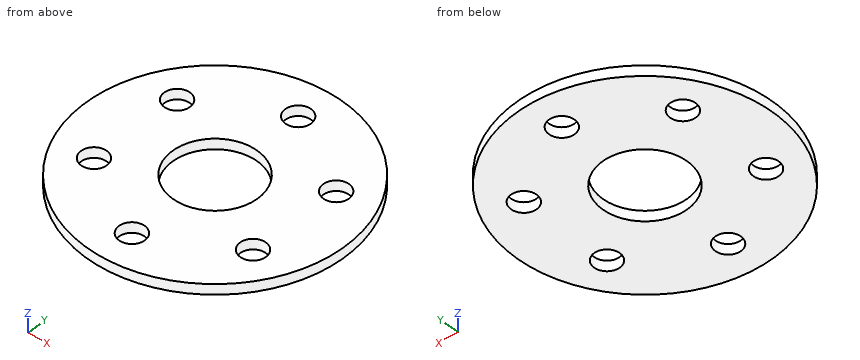
```python
from build123d import *

# Parameters (mm, degrees)
SKETCH1_R           = 25
SKETCH1_R_2         = 8.25
SKETCH1_R_3         = 2.5
BOSS_EXTRUDE1_DEPTH = 1


with BuildPart() as part:
    # Sketch1 (on Front Plane) → Boss-Extrude1 (new, symmetric)
    with BuildSketch(Plane.XY):
        Circle(SKETCH1_R)
        Circle(SKETCH1_R_2, mode=Mode.SUBTRACT)
        with Locations((0, 18)):
            Circle(SKETCH1_R_3, mode=Mode.SUBTRACT)
        with Locations((15.588457268, 9)):
            Circle(SKETCH1_R_3, mode=Mode.SUBTRACT)
        with Locations((15.588457268, -9)):
            Circle(SKETCH1_R_3, mode=Mode.SUBTRACT)
        with Locations((0, -18)):
            Circle(SKETCH1_R_3, mode=Mode.SUBTRACT)
        with Locations((-15.588457268, -9)):
            Circle(SKETCH1_R_3, mode=Mode.SUBTRACT)
        with Locations((-15.588457268, 9)):
            Circle(SKETCH1_R_3, mode=Mode.SUBTRACT)
    extrude(amount=BOSS_EXTRUDE1_DEPTH, both=True)


solid = part.part
```
Build history of the part. All positions in model axes, mm. Round coordinates to 2 decimals unless told otherwise and drop trailing zeros. Loops run counter-clockwise (first coordinate to the right, second up) from the corner with the lowest first, then second, coordinate; pieces in that order, holes last.
Item 1: Saw through at B-B (x = 0). List the corners of the cut face in (y, z), then the cut area to 3 significant figures.
Item 2: Saw through at C-C (x = -5). List the corners of the cut face in (y, z).
Item 3: Saw through at D-D (y = -9). List the corners of the cut face in (x, z), then the cut area to 3 significant figures.
Item 4: Saw through at A-A (y = 0). List the corners of the cut face in (x, z).
Item 5: Drill centre lines: line 1 along Y through (x, z) = (0, -0.4); line 2 along X through (y, z) = (-17.5, 0.55); line 3 along Y through (x, z) = (-5, 0.25). Where is each one in solid material? Low to high.
Worked answers:
1. outline: (-25, -1) - (-20.5, -1) - (-20.5, 1) - (-25, 1) - close; (-15.5, -1) - (-8.25, -1) - (-8.25, 1) - (-15.5, 1) - close; (8.25, -1) - (15.5, -1) - (15.5, 1) - (8.25, 1) - close; (20.5, -1) - (25, -1) - (25, 1) - (20.5, 1) - close
1. area: 47.0 mm2
2. outline: (-24.49, -1) - (-6.56, -1) - (-6.56, 1) - (-24.49, 1) - close; (6.56, -1) - (24.49, -1) - (24.49, 1) - (6.56, 1) - close
3. outline: (-23.32, -1) - (-18.09, -1) - (-18.09, 1) - (-23.32, 1) - close; (-13.09, -1) - (13.09, -1) - (13.09, 1) - (-13.09, 1) - close; (18.09, -1) - (23.32, -1) - (23.32, 1) - (18.09, 1) - close
3. area: 73.3 mm2
4. outline: (-25, -1) - (-8.25, -1) - (-8.25, 1) - (-25, 1) - close; (8.25, -1) - (25, -1) - (25, 1) - (8.25, 1) - close
5. line 1: y = -25 to -20.5, -15.5 to -8.25, 8.25 to 15.5, 20.5 to 25
5. line 2: x = -17.85 to -2.45, 2.45 to 17.85
5. line 3: y = -24.49 to -6.56, 6.56 to 24.49
